For this review, take the finished solid that the model builds, in its own axes (mm). A direction names the side the tool comes from. Round coordinates to 2 decimals unless told otherwise and drop trailing zeros. Order: outer loops, then holes, each group sorted by start corner. A loop starts at its lowest first (then second) coordinate and runs counter-clockwise, first axis right, second up. Notation, with made-up numbers: (87, -12.5) -> (101, -12.5) arc R25 cw to (101, 18.5) -> close; hole circle Ø6 at (11, 1.5). An arc over 180 degrees is marked (long way). Use a Markdown table: item, result. Add a question column.
1) Consider section A-A (y = -4.5). State the section outline as (x, z) points, plus the area to 3 significant figures.
2) Draft analysis for pull direction Z (two halves, no side actions). For faces 4 (the face through (1, 0, 1)), 5 (the face through (0, 0.4, 0)), 6 (the face through (-1.9, 0.2, -0.08)), state which applies: pulls with the +Z half, pulls with the -Z half, needs draft (parallel to the pull), parting line crosses it, or undercut.
3) Machinability: for faces 1 (the face through (-0.75, 1, 0)), 2 (the face through (0, -6, 0)), 3 (the face through (-0.95, -2.86, 0.04)), which of the approach directions +Z, -Z, +X, -X, +Y, -Y give a long, thin tool a straight path to every point of the face, cutting with its end or side? Answer none if there is none.
4) Wall thickness on line 1 along X through (y, z) = (1.25, 0.15); line 2 along Y through (x, z) = (-0.35, 0.05); line 3 along Z through (x, y) = (-0.6, -4): over which ranges is each line inside the solid? List them lowest first. Write a range as [from, to].
5) Clearance check with flat-ended pins moving along their axes: P1, Ø2, axis at y = -0.5, z = -1, coming from the -X side; P2, Ø1.5, axis at x = -1, y = -3, coming from the +Z side; P3, Ø1, axis at x = -1, y = -2.5, coming from the +Z side. State where each tip first meets the part, or that it passes through.
```python
from build123d import *

# Parameters (mm, degrees)
SKETCH_1_R          = 1.9
EXTRUDE_1_DEPTH     = 1.4
CUT_EXTRUDE_1_DEPTH = 1
FILLET_1_R          = 1
SKETCH_3_R          = 0.95
EXTRUDE_2_DEPTH     = 6
CHAMFER_1_SIZE      = 0.2


with BuildPart() as part:
    # 草图1 → 凸台-拉伸1 (new body)
    with BuildSketch(Plane(origin=(0, 0, 0), x_dir=(1, 0, 0), z_dir=(0, 1, 0))):
        Circle(SKETCH_1_R)
    extrude(amount=EXTRUDE_1_DEPTH)

    # 草图2 → 切除-拉伸1 (cut)
    with BuildSketch(Plane(origin=(0, 1.4, 0), x_dir=(1, 0, 0), z_dir=(0, 1, 0))):
        Polygon((0, -0.866025404), (0.75, -0.433012702), (0.75, 0.433012702), (0, 0.866025404), (-0.75, 0.433012702), (-0.75, -0.433012702), align=None)
    extrude(amount=-CUT_EXTRUDE_1_DEPTH, mode=Mode.SUBTRACT)

    # 圆角1
    fillet_1_edges = [part.edges().sort_by_distance(p)[0] for p in [
        (-1.9, 1.4, 0),
    ]]
    fillet(fillet_1_edges, radius=FILLET_1_R)

    # 草图3 → 凸台-拉伸2 (add)
    with BuildSketch(Plane.XZ):
        Circle(SKETCH_3_R)
    extrude(amount=EXTRUDE_2_DEPTH)

    # 倒角1
    chamfer_1_edges = [part.edges().sort_by_distance(p)[0] for p in [
        (-0.95, -6, 0),
    ]]
    chamfer(chamfer_1_edges, length=CHAMFER_1_SIZE)


solid = part.part
```
Results list:
| question | item | result |
|---|---|---|
| 1 | outline | circle Ø1.9 at (0, 0) |
| 1 | area | 2.84 mm2 |
| 2 | face 4 | needs draft |
| 2 | face 5 | undercut |
| 2 | face 6 | parting line crosses it |
| 3 | face 1 | +Y |
| 3 | face 2 | +Z, -Z, +X, -X, -Y |
| 3 | face 3 | -Y |
| 4 | line 1 | [-1.42, -0.75], [0.75, 1.42] |
| 4 | line 2 | [-6, 0.4] |
| 4 | line 3 | [-0.74, 0.74] |
| 5 | P1 | x = -1.9 |
| 5 | P2 | z = 0.92 |
| 5 | P3 | z = 0.81 |
